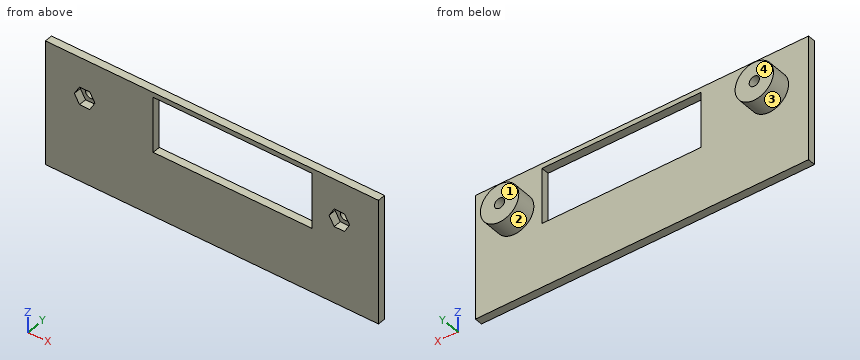
```python
from build123d import *

# Parameters (mm, degrees)
SKETCH1_W             = 170
SKETCH1_H             = 64
SKETCH1_R             = 10
SKETCH1_W_2           = 81
SKETCH1_H_2           = 28.5
BOSS_EXTRUDE1_DEPTH   = 4
BOSS_EXTRUDE2_START   = -4
SKETCH2_R             = 10
SKETCH2_R_2           = 9.8
BOSS_EXTRUDE2_DEPTH   = 4
SKETCH3_R             = 9.8
BOSS_EXTRUDE3_DEPTH   = 10
BOSS_EXTRUDE3_2_DEPTH = 10
BOSS_EXTRUDE4_START   = 4
SKETCH4_R             = 9.8
SKETCH4_R_2           = 2.6
BOSS_EXTRUDE4_DEPTH   = 4
SKETCH5_R             = 2.6
CUT_EXTRUDE1_DEPTH    = 47


with BuildPart() as part:
    # Sketch1 → Boss-Extrude1 (new body)
    with BuildSketch(Plane(origin=(0, 0, 0), x_dir=(1, 0, 0), z_dir=(0, 1, 0))):
        with Locations((85, 32)):
            Rectangle(SKETCH1_W, SKETCH1_H)
        with Locations(Location((20, 20, 0), (0, 0, 270))):
            Circle(SKETCH1_R, mode=Mode.SUBTRACT)
        with Locations(Location((150, 20, 0), (0, 0, 270))):
            Circle(SKETCH1_R, mode=Mode.SUBTRACT)
        with Locations((95.5, 16.75)):
            Rectangle(SKETCH1_W_2, SKETCH1_H_2, mode=Mode.SUBTRACT)
    extrude(amount=BOSS_EXTRUDE1_DEPTH)

    # Sketch2 → Boss-Extrude2 (add)
    # profile 1 of 2: a face of its own
    with BuildSketch(Plane(origin=(0, 4, 0), x_dir=(1, 0, 0), z_dir=(0, 1, 0)).offset(BOSS_EXTRUDE2_START)):
        with Locations((20, 20)):
            Circle(SKETCH2_R)
        with Locations(Location((20, 20, 0), (0, 0, 270))):
            Circle(SKETCH2_R_2, mode=Mode.SUBTRACT)
    # profile 2 of 2: a face of its own
    with BuildSketch(Plane(origin=(0, 4, 0), x_dir=(1, 0, 0), z_dir=(0, 1, 0)).offset(BOSS_EXTRUDE2_START)):
        with Locations((150, 20)):
            Circle(SKETCH2_R)
        with Locations(Location((150, 20, 0), (0, 0, 270))):
            Circle(SKETCH2_R_2, mode=Mode.SUBTRACT)
    extrude(amount=BOSS_EXTRUDE2_DEPTH)



with BuildPart() as body_2:
    # Sketch3 → Boss-Extrude3 (new body)
    with BuildSketch(Plane(origin=(0, 4, 0), x_dir=(1, 0, 0), z_dir=(0, 1, 0))):
        with Locations(Location((20, 20, 0), (0, 0, 270))):
            Circle(SKETCH3_R)
    extrude(amount=BOSS_EXTRUDE3_DEPTH)


with BuildPart() as body_3:
    # Sketch3 → Boss-Extrude3 2 (new body)
    with BuildSketch(Plane(origin=(0, 4, 0), x_dir=(1, 0, 0), z_dir=(0, 1, 0))):
        with Locations(Location((150, 20, 0), (0, 0, 270))):
            Circle(SKETCH3_R)
    extrude(amount=BOSS_EXTRUDE3_2_DEPTH)


with BuildPart() as part_1:
    add(part.part)

    add(body_2.part)  # Boss-Extrude4 merges body 2

    add(body_3.part)  # Boss-Extrude4 merges body 3
    # Sketch4 → Boss-Extrude4 (add)
    # profile 1 of 4: a face of its own
    with BuildSketch(Plane.XZ.offset(-4).offset(BOSS_EXTRUDE4_START)):
        with Locations(Location((20, -20, 0), (0, 0, 90))):
            Circle(SKETCH4_R)
        Polygon((25.25388745, -20), (22.626943725, -15.45), (17.373056275, -15.45), (14.74611255, -20), (17.373056275, -24.55), (22.626943725, -24.55), align=None, mode=Mode.SUBTRACT)
    # profile 2 of 4: a face of its own
    with BuildSketch(Plane.XZ.offset(-4).offset(BOSS_EXTRUDE4_START)):
        with Locations(Location((20, -20, 0), (0, 0, 90))):
            Circle(SKETCH4_R_2)
    # profile 3 of 4: a face of its own
    with BuildSketch(Plane.XZ.offset(-4).offset(BOSS_EXTRUDE4_START)):
        with Locations(Location((150, -20, 0), (0, 0, 90))):
            Circle(SKETCH4_R)
        Polygon((155.25388745, -20), (152.626943725, -15.45), (147.373056275, -15.45), (144.74611255, -20), (147.373056275, -24.55), (152.626943725, -24.55), align=None, mode=Mode.SUBTRACT)
    # profile 4 of 4: a face of its own
    with BuildSketch(Plane.XZ.offset(-4).offset(BOSS_EXTRUDE4_START)):
        with Locations(Location((150, -20, 0), (0, 0, 90))):
            Circle(SKETCH4_R_2)
    extrude(amount=-BOSS_EXTRUDE4_DEPTH)

    # Sketch5 → Cut-Extrude1 (cut)
    with BuildSketch(Plane.XZ):
        with Locations(Location((20, -20, 0), (0, 0, 90))):
            Circle(SKETCH5_R)
        with Locations(Location((150, -20, 0), (0, 0, 90))):
            Circle(SKETCH5_R)
    extrude(amount=-CUT_EXTRUDE1_DEPTH, mode=Mode.SUBTRACT)


solid = part_1.part
```
Geometry: final body of the model. Coordinates: model frame, mm. Face numbers are marked on the shaded views. A direction names the side the tool comes from. Give positions to 0.01 mm unless a question says otherwise; leave off trailing zeros. Loops run counter-clockwise (first coordinate to the right, second up) from the corner with the lowest first, then second, coordinate; pieces in that order, holes last. Notation, with made-up numbers: (14, 61) -> (72, 61) arc R27 cw to (72, 86) -> close; hole circle Ø10 at (69, 58). An arc over 180 degrees is marked (long way). Use one line per item in the form item = value.
Item 1: Section query B-B on y = 10.5. Output: boundary loops of the cut face in (x, z), and give its area (3 significant figures).
A:
outline = circle Ø19.6 at (20, -20); circle Ø19.6 at (150, -20); hole circle Ø5.2 at (20, -20); hole circle Ø5.2 at (150, -20)
area = 561 mm^2
Item 2: Section query A-A on x = 131. Output: boundary loops of the cut face in (y, z).
A:
outline = (0, -64) -> (4, -64) -> (4, -31) -> (0, -31) -> close; (0, -2.5) -> (4, -2.5) -> (4, 0) -> (0, 0) -> close
Item 3: Section query D-D on z = -44. Output: boundary loops of the cut face in (x, y).
A:
outline = (0, 0) -> (170, 0) -> (170, 4) -> (0, 4) -> close
Item 4: Line query: probe 1 along X at (y, z) = (7.5, -20); probe 2 along Y at (x, z) = (86.5, -36); probe 3 along Z at (x, y) = (22, 7). Output: solid intervals per line, ascending.
A:
probe_1 = 10.2 to 17.4, 22.6 to 29.8, 140.2 to 147.4, 152.6 to 159.8
probe_2 = 0 to 4
probe_3 = -29.59 to -21.66, -18.34 to -10.41
Item 5: Access query for the marked faces 3 and 4. Directions: +Z, -Z, +X, -X, +Y, -Y. A direction counts if a zero-diameter tool reaches every point of the face in a straight line with its end or side. Return the directions, or none.
A:
face_3 = +Y
face_4 = +Z, -Z, +X, -X, +Y
Item 6: Section query C-C on x = 20. Output: boundary loops of the cut face in (y, z).
A:
outline = (0, -64) -> (4, -64) -> (4, -29.8) -> (14, -29.8) -> (14, -22.6) -> (4, -22.6) -> (4, -24.55) -> (0, -24.55) -> close; (0, -15.45) -> (4, -15.45) -> (4, -17.4) -> (14, -17.4) -> (14, -10.2) -> (4, -10.2) -> (4, 0) -> (0, 0) -> close
Item 7: Pin query (flat end, axial travel): P1, Ø1, axis at x = 151.5, y = 10.5, coming from the -Z side; P2, Ø2.5, axis at x = 19, z = -19, coming from the -Y side; P3, Ø3, axis at x = 69.5, z = -35, coming from the +Y side. Return the tip coordinate at first contact, or that it passes through.
A:
P1 = -29.75
P2 = 4
P3 = 4
Item 8: Draft query along X for the marked faces 1 and 2. Return one class per face: pulls with the +X half, pulls with the -X half, needs draft (parallel to the pull), parting line crosses it, or undercut.
A:
face_1 = needs draft
face_2 = undercut
